Design review of the part built by this model. Coordinates are the model's own, in mm. Round coordinates to 2 decimals unless told otherwise and drop trailing zeros. Loops run counter-clockwise (first coordinate to the right, second up) from the corner with the lowest first, then second, coordinate; pieces in that order, holes last. Notation, with made-up numbers: (8, 17) -> (41, 17) arc R19 ccw to (41, 34) -> close; hole circle Ø11 at (-17, 36). An arc over 180 degrees is marked (long way). Answer as CSV lines item,"result". Start each with the question number.
(1) For P1, Ø6, axis at x = -3, y = -5.5, coming from the +Z side; P2, Ø1, axis at y = -2.5, z = 5, coming from the -X side; P3, Ø8, axis at x = 17, y = -10.5, coming from the -Z side; P4, Ø1, axis at y = 9, z = 1.5, coming from the +X side, all flat-tipped, find the tip position at first contact; note any pin that passes through.
(2) Draft analysis for pull direction Y (two halves, no side actions). For faces 1 (the face through (6, 10, 7)), 2 (the face through (32.973, 9.444, 3.451)), 3 (the face through (-16.269, 3.364, 3.451)), 4 (the face through (0, -13.2, 4)), state which applies: +Y half, -Y half, draft (parallel to the pull), parting line (faces both ways), or undercut.
(3) To check wall thickness, follow line 1 (X direction, y = 5.75, z = 1.25); line 2 (X direction, y = 0.5, z = 6.5); line 3 (Y direction, x = -26.5, z = 3.25). State the ranges of each line that lie inside material, in increasing order. Write a range as from..to.
(4) Take a section at A-A, the plane z = 5. Write out the cut boundary in (x, y).
(5) Take a section at C-C, the plane x = 0. Write out the cut boundary in (y, z).
(6) Take a section at D-D, the plane x = 18. Write out the cut boundary in (y, z), and give its area (3 significant figures).
(7) Take a section at B-B, the plane y = 0. Write out the cut boundary in (x, z), and give its area (3 significant figures).
from build123d import *

# Parameters (mm, degrees)
F0_R     = 11.2
F1_DEPTH = 7
F2_R     = 1.5


with BuildPart() as f1:
    # F0 (on Top) → F1 (new body)
    with BuildSketch(Plane.XY):
        with BuildLine():
            Line((0, 13.2), (-26.95201, 13.2))
            ThreePointArc((-26.95201, 13.2), (-40.15201, 0), (-26.95201, -13.2))
            Line((-26.95201, -13.2), (0, -13.2))
            Line((0, -13.2), (26.95201, -13.2))
            ThreePointArc((26.95201, -13.2), (40.15201, 0), (26.95201, 13.2))
            Line((26.95201, 13.2), (0, 13.2))
        make_face()
        with Locations((-26.95201, 0)):
            Circle(F0_R, mode=Mode.SUBTRACT)
        Circle(F0_R, mode=Mode.SUBTRACT)
        with Locations((26.95201, 0)):
            Circle(F0_R, mode=Mode.SUBTRACT)
    extrude(amount=F1_DEPTH)

    # F2
    f2_edges = [f1.edges().sort_by_distance(p)[0] for p in [
        (0, 13.2, 0),
        (-40.15201, 0, 0),
        (0, -13.2, 0),
        (40.15201, 0, 0),
    ]]
    fillet(f2_edges, radius=F2_R)


solid = f1.part
The answers:
1,P1,"through"
1,P2,"x = -40"
1,P3,"z = 0"
1,P4,"x = 37.05"
2,face 1,"draft"
2,face 2,"undercut"
2,face 3,"undercut"
2,face 4,"-Y half"
3,line 1,"-38.81..-36.56, -17.34..-9.61, 9.61..17.34, 36.56..38.81"
3,line 2,"-40.14..-38.14, -15.76..-11.19, 11.19..15.76, 38.14..40.14"
3,line 3,"-13.2..-11.19, 11.19..13.2"
4,outline,"(-26.95, -13.2) -> (26.95, -13.2) arc R13.2 ccw to (26.95, 13.2) -> (-26.95, 13.2) arc R13.2 ccw to start; hole circle Ø22.4 at (-26.95, 0); hole circle Ø22.4 at (0, 0); hole circle Ø22.4 at (26.95, 0)"
5,outline,"(-13.2, 1.5) arc R1.5 ccw to (-11.7, 0) -> (-11.2, 0) -> (-11.2, 7) -> (-13.2, 7) -> close; (11.2, 0) -> (11.7, 0) arc R1.5 ccw to (13.2, 1.5) -> (13.2, 7) -> (11.2, 7) -> close"
6,outline,"(-13.2, 1.5) arc R1.5 ccw to (-11.7, 0) -> (-6.73, 0) -> (-6.73, 7) -> (-13.2, 7) -> close; (6.73, 0) -> (11.7, 0) arc R1.5 ccw to (13.2, 1.5) -> (13.2, 7) -> (6.73, 7) -> close"
6,area,"89.6 mm²"
7,outline,"(-40.15, 1.5) arc R1.5 ccw to (-38.65, 0) -> (-38.15, 0) -> (-38.15, 7) -> (-40.15, 7) -> close; (-15.75, 0) -> (-11.2, 0) -> (-11.2, 7) -> (-15.75, 7) -> close; (11.2, 0) -> (15.75, 0) -> (15.75, 7) -> (11.2, 7) -> close; (38.15, 0) -> (38.65, 0) arc R1.5 ccw to (40.15, 1.5) -> (40.15, 7) -> (38.15, 7) -> close"
7,area,"90.8 mm²"
